For this review, take the finished solid that the model builds, in its own axes (mm). Face numbers are marked on the shaded views. A direction names the side the tool comes from. Give positions to 0.01 mm unless a question says otherwise; leave off trailing zeros. Write each loop counter-clockwise with the first axis right and the second up, starting at its lowest first coordinate (ties: lowest second). Pieces come first, ordered by that corner, then holes. Notation, with made-up numbers: M 59,33.5 L 84,33.5 A16 ccw 84,44.5 Z; hole C 11,73 d9. An arc over 180 degrees is marked long. Write item = value, one per line.
```python
from build123d import *

# Parameters (mm, degrees)
SKETCH2_W          = 3.25
SKETCH2_H          = 3.25
CUT_EXTRUDE1_DEPTH = 40
CHAMFER1_SIZE      = 1
SKETCH3_W          = 3.25
SKETCH3_H          = 3.25
CUT_EXTRUDE2_DEPTH = 22


with BuildPart() as part:
    # Sketch1 → Revolve1 (revolve)
    with BuildSketch(Plane.XY, mode=Mode.PRIVATE) as revolve1_sk:
        Polygon((0, 0), (7.5, 0), (7.5, 15), (10, 15), (10, 55), (15, 55), (15, 77), (9, 77), (9, 99), (7.5, 99), (7.5, 103), (0, 103), align=None)
    revolve(revolve1_sk.sketch.rotate(Axis((0, 103, 0), (0, -1, 0)), 90), axis=Axis((0, 103, 0), (0, -1, 0)))

    # Sketch2 → Cut-Extrude1 (cut)
    with BuildSketch(Plane.XZ.offset(-15)):
        with Locations((0, 10)):
            Rectangle(SKETCH2_W, SKETCH2_H)
    extrude(amount=-CUT_EXTRUDE1_DEPTH, mode=Mode.SUBTRACT)

    # Chamfer1
    chamfer1_edges = [part.edges().sort_by_distance(p)[0] for p in [
        (0, 77, -15),
        (0, 55, -15),
        (0, 15, -10),
        (0, 0, -7.5),
        (0, 103, -7.5),
        (0, 99, -9),
    ]]
    chamfer(chamfer1_edges, length=CHAMFER1_SIZE)

    # Sketch3 → Cut-Extrude2 (cut)
    with BuildSketch(Plane(origin=(0, 99, 0), x_dir=(1, 0, 0), z_dir=(0, 1, 0))):
        with Locations((0, 9)):
            Rectangle(SKETCH3_W, SKETCH3_H)
    extrude(amount=-CUT_EXTRUDE2_DEPTH, mode=Mode.SUBTRACT)


solid = part.part
```
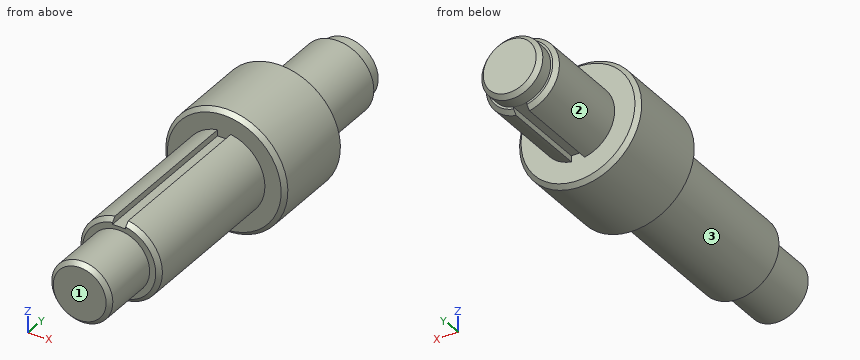
1. We need section C-C, the plane y = 86. Write out the cut boundary in (x, z) (3 decimals), then the cut area to 3 significant figures.
Responses:
outline = M -1.625,-8.852 L -1.625,-7.375 L 1.625,-7.375 L 1.625,-8.852 A9 ccw long Z
area = 249 mm2
2. Machinability: for the marked faces 1, 2 and 3, which of the approach directions +Z, -Z, +X, -X, +Y, -Y give a long, thin tool a straight path to every point of the face, cutting with its end or side? Answer none if there is none.
Responses:
face_1 = +Z, -Z, +X, -X, -Y
face_2 = +Y
face_3 = -Y
3. For line 1 along Y through (x, z) = (-11, -7.5); line 2 along X through (y, z) = (68.5, 0.5); line 3 along X through (y, z) = (41, 0.25), list the stretches that pass through material, from the lowest coordinate up. Write a range as from..to.
Responses:
line_1 = 55..77
line_2 = -14.99..14.99
line_3 = -10..10
4. Insertion check: P1, Ø4, axis at x = 3.5, y = 92, coming from the -Z side; P2, Ø1, axis at x = 0, y = 34.5, coming from the +Z side (3 decimals); P3, Ø2, axis at x = -7.5, z = 1.5, coming from the +Y side; P4, Ø6, axis at x = 3.5, z = 4, coming from the -Y side. Each pin has a flat end and moves straight along its axis. Give the tip position at first contact, or say it passes through.
Responses:
P1 = -8.85
P2 = 8.375
P3 = 102.85
P4 = 0
